from build123d import *

# Parameters (mm, degrees)
SKETCH1_W           = 28
SKETCH1_H           = 15.75
SKETCH1_W_2         = 6
SKETCH1_H_2         = 3
BOSS_EXTRUDE1_DEPTH = 1
CUT_EXTRUDE1_REACH  = 18.094
SKETCH2_R           = 1.475
SKETCH5_W           = 28
SKETCH5_H           = 15.75
SKETCH5_W_2         = 6
SKETCH5_H_2         = 3
BOSS_EXTRUDE4_DEPTH = 0.5
SKETCH3_R           = 2.475
SKETCH3_R_2         = 1.475
BOSS_EXTRUDE2_DEPTH = 1
SKETCH4_W           = 28
SKETCH4_H           = 15.75
SKETCH4_W_2         = 26
SKETCH4_H_2         = 13.75
BOSS_EXTRUDE3_DEPTH = 3.5
FILLET1_R           = 2


with BuildPart() as part:
    # Sketch1 → Boss-Extrude1 (new body)
    with BuildSketch(Plane.XY):
        Rectangle(SKETCH1_W, SKETCH1_H)
        with Locations((0, -2.285)):
            Rectangle(SKETCH1_W_2, SKETCH1_H_2, mode=Mode.SUBTRACT)
    extrude(amount=BOSS_EXTRUDE1_DEPTH)

    # Sketch2 → Cut-Extrude1 (cut, up to next)
    with BuildSketch(Plane.XY.offset(1), mode=Mode.PRIVATE) as cut_extrude1_sk1:
        with Locations((10, 0)):
            Circle(SKETCH2_R)
    cut_extrude1_tool1 = extrude(cut_extrude1_sk1.sketch, amount=-CUT_EXTRUDE1_REACH, mode=Mode.PRIVATE) & part.part
    # Sketch2 → Cut-Extrude1 (cut, up to next)
    with BuildSketch(Plane.XY.offset(1), mode=Mode.PRIVATE) as cut_extrude1_sk2:
        with Locations((-10, 0)):
            Circle(SKETCH2_R)
    cut_extrude1_tool2 = extrude(cut_extrude1_sk2.sketch, amount=-CUT_EXTRUDE1_REACH, mode=Mode.PRIVATE) & part.part
    add(cut_extrude1_tool1.solids().sort_by_distance((10, 0, 1))[0], mode=Mode.SUBTRACT)
    add(cut_extrude1_tool2.solids().sort_by_distance((-10, 0, 1))[0], mode=Mode.SUBTRACT)

    # Sketch5 → Boss-Extrude4 (add)
    with BuildSketch(Plane.XY.offset(1)):
        Rectangle(SKETCH5_W, SKETCH5_H)
        with Locations((0, -2.285)):
            Rectangle(SKETCH5_W_2, SKETCH5_H_2, mode=Mode.SUBTRACT)
    extrude(amount=BOSS_EXTRUDE4_DEPTH)

    # Sketch3 → Boss-Extrude2 (add)
    # profile 1 of 2: a face of its own
    with BuildSketch(Plane(origin=(0, 0, 0), x_dir=(-1, 0, 0), z_dir=(0, 0, -1))):
        with Locations(Location((-10, 0, 0), (0, 0, 180))):
            Circle(SKETCH3_R)
        with Locations(Location((-10, 0, 0), (0, 0, 180))):
            Circle(SKETCH3_R_2, mode=Mode.SUBTRACT)
    # profile 2 of 2: a face of its own
    with BuildSketch(Plane(origin=(0, 0, 0), x_dir=(-1, 0, 0), z_dir=(0, 0, -1))):
        with Locations(Location((10, 0, 0), (0, 0, 180))):
            Circle(SKETCH3_R)
        with Locations(Location((10, 0, 0), (0, 0, 180))):
            Circle(SKETCH3_R_2, mode=Mode.SUBTRACT)
    extrude(amount=BOSS_EXTRUDE2_DEPTH)

    # Sketch4 → Boss-Extrude3 (add)
    with BuildSketch(Plane(origin=(0, 0, 0), x_dir=(-1, 0, 0), z_dir=(0, 0, -1))):
        Rectangle(SKETCH4_W, SKETCH4_H)
        Rectangle(SKETCH4_W_2, SKETCH4_H_2, mode=Mode.SUBTRACT)
    extrude(amount=BOSS_EXTRUDE3_DEPTH)

    # Fillet1
    fillet1_edges = [part.edges().sort_by_distance(p)[0] for p in [
        (0, -7.875, 1.5),
        (14, 0, 1.5),
        (0, 7.875, 1.5),
        (-14, 0, 1.5),
        (14, -7.875, -1),
        (-14, -7.875, -1),
        (-14, 7.875, -1),
        (14, 7.875, -1),
    ]]
    fillet(fillet1_edges, radius=FILLET1_R)


solid = part.part
Verification items for the finished model (mm, model axes). A direction names the side the tool comes from. Coordinates: 2 decimals unless noted, no trailing zeros. Write each loop counter-clockwise with the first axis right and the second up, starting at its lowest first coordinate (ties: lowest second). Pieces come first, ordered by that corner, then holes. Notation, with made-up numbers: M 1,0.25 L 34,0.25 A23 ccw 34,12.25 Z; hole C 4,26 d5. An arc over 180 degrees is marked long. Use a Markdown table: item, result.
Q1. Sectioned sample at A-A, the plane z = -2.6. Record the boundary of the cut face in (x, y) (3 decimals), plus the area to 3 significant figures.
Reply:
| item | result |
|---|---|
| outline | M -14,-5.875 A2 ccw -12,-7.875 L 12,-7.875 A2 ccw 14,-5.875 L 14,5.875 A2 ccw 12,7.875 L -12,7.875 A2 ccw -14,5.875 Z; hole M -13,-6.875 L 13,-6.875 L 13,6.875 L -13,6.875 Z |
| area | 80.1 mm² |
Q2. Go/stop test with flat-tipped pins: P1, Ø3, axis at y = 4, z = 0, coming from the +X side; P2, Ø0.8, axis at y = -1.5, z = 1, coming from the +X side; P3, Ø1.5, axis at x = -7, y = 5, coming from the -Z side; P4, Ø1.6, axis at x = 1, z = 0.5, coming from the -Y side (3 decimals). Record where each tip stops, or that it passes through.
Reply:
| item | result |
|---|---|
| P1 | stops at x = 14 |
| P2 | stops at x = 13.67 |
| P3 | stops at z = 0 |
| P4 | stops at y = -7.865 |
Q3. Thickness scan on line 1 (Y direction, x = 9, z = -2.5) (3 decimals); line 2 (X direction, y = -1.5, z = -2.8); line 3 (X direction, y = 0, z = 0.45) (3 decimals). Record the ranges inside material, lowest first.
Reply:
| item | result |
|---|---|
| line 1 | y = -7.875 to -6.875, 6.875 to 7.875 |
| line 2 | x = -14 to -13, 13 to 14 |
| line 3 | x = -13.76 to -11.475, -8.525 to 8.525, 11.475 to 13.76 |
Q4. Sectioned sample at C-C, the plane y = 4.5. Record the boundary of the cut face in (x, z), plus the area to 3 significant figures.
Reply:
| item | result |
|---|---|
| outline | M -14,-3.5 L -13,-3.5 L -13,0 L 13,0 L 13,-3.5 L 14,-3.5 L 14,-0.5 A2 ccw 12,1.5 L -12,1.5 A2 ccw -14,-0.5 Z |
| area | 47.3 mm² |
Q5. Sectioned sample at D-D, the plane z = 0.5. Record the boundary of the cut face in (x, y) (3 decimals), plus the area to 3 significant figures.
Reply:
| item | result |
|---|---|
| outline | M -13.732,-5.875 A1.732 ccw -12,-7.607 L 12,-7.607 A1.732 ccw 13.732,-5.875 L 13.732,5.875 A1.732 ccw 12,7.607 L -12,7.607 A1.732 ccw -13.732,5.875 Z; hole C -10,0 d2.95; hole M -3,-3.785 L 3,-3.785 L 3,-0.785 L -3,-0.785 Z; hole C 10,0 d2.95 |
| area | 384 mm² |
Q6. Sectioned sample at B-B, the plane x = -4. Record the boundary of the cut face in (y, z) (3 decimals), plus the area to 3 significant figures.
Reply:
| item | result |
|---|---|
| outline | M -7.875,-3.5 L -6.875,-3.5 L -6.875,0 L 6.875,0 L 6.875,-3.5 L 7.875,-3.5 L 7.875,-0.5 A2 ccw 5.875,1.5 L -5.875,1.5 A2 ccw -7.875,-0.5 Z |
| area | 28.9 mm² |
Q7. Set-up check for faces 1 (the face through (13.43, -7.274, -2.021)), 2 (the face through (-3, -2, 1)), 3 (the face through (0, -6.875, -2)): record each of +Z, -Z, +X, -X, +Y, -Y from which the full face is reachable in a straight line by a thin tool's end or side.
Reply:
| item | result |
|---|---|
| face 1 | +Z, -Z, +X, -Y |
| face 2 | +Z, -Z |
| face 3 | -Z |
Q8. Draft check along X on faces 4 (the face through (13, 0, -2)), 5 (the face through (13.43, 0.08, 0.9)), 6 (the face through (-13.43, 0.08, 0.9)), 7 (the face through (0, 7.875, -2)). Enter one of: +X half, -X half, draft (parallel to the pull), parting line (faces both ways), or undercut.
Reply:
| item | result |
|---|---|
| face 4 | undercut |
| face 5 | +X half |
| face 6 | -X half |
| face 7 | draft |
